Build history of the part. All positions in model axes, mm. Face numbers are marked on the shaded views. A direction names the side the tool comes from. Round coordinates to 2 decimals unless told otherwise and drop trailing zeros. Write each loop counter-clockwise with the first axis right and the second up, starting at its lowest first coordinate (ties: lowest second). Pieces come first, ordered by that corner, then holes. Notation, with made-up numbers: (17, 9) -> (41, 9) arc R9 ccw to (41, 18) -> close; hole circle Ø6 at (-3.5, 55). An arc over 180 degrees is marked (long way). Return JSON: item names as keys, results as strings.
from build123d import *


with BuildPart() as f1:
    # F0 (on Right) → F1 (revolve)
    with BuildSketch(Plane.YZ):
        with BuildLine():
            Line((-123.77214, 15), (-123.77214, 0))
            Line((-123.77214, 0), (96.22786, 0))
            Line((96.22786, 0), (96.22786, 15))
            Line((96.22786, 15), (78.22786, 15))
            ThreePointArc((78.22786, 15), (73.278113, 17.050253), (71.22786, 22))
            Line((71.22786, 22), (71.22786, 24.047213))
            ThreePointArc((71.22786, 24.047213), (69.177608, 28.996961), (64.22786, 31.047213))
            Line((64.22786, 31.047213), (-23.778022, 31.047213))
            ThreePointArc((-23.778022, 31.047213), (-33.246551, 21.403982), (-43.675041, 30))
            Line((-43.675041, 30), (-108.77214, 30))
            ThreePointArc((-108.77214, 30), (-119.378742, 25.606602), (-123.77214, 15))
        make_face()
    revolve(axis=Axis((0, 76.22786, 0), (0, 1, 0)))


solid = f1.part
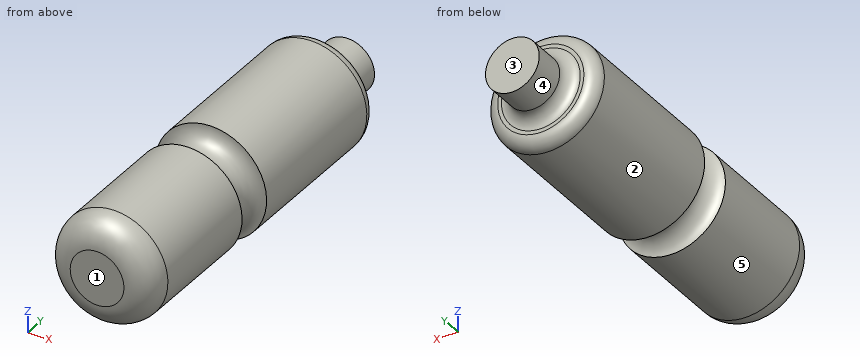
Q1. Saw through at D-D on y = -1.5. List the corners of the cut face in (x, z).
Verdict:
{"outline": "circle Ø62.09 at (0, 0)"}
Q2. Two-plate mould, pull along Z, no slides. Class the marked faces 1 and 2: +Z half, -Z half, draft (parallel to the pull), parting line (faces both ways), or undercut.
Verdict:
{"face 1": "draft", "face 2": "parting line"}
Q3. Pin check, flat tips, straight feed: pin 1 Ø1.5 at (x, y) = (-3, 31.5) entering from +Z; pin 2 Ø6 at (x, y) = (-15.5, -46.5) entering from +Z; pin 3 Ø6 at (y, z) = (16, -23.5) entering from +X. Stop position of each tip, or through.
Verdict:
{"pin 1": "stops at z = 30.97", "pin 2": "stops at z = 27.27", "pin 3": "stops at x = 23.32"}
Q4. Saw through at C-C on y = -106. List the corners of the cut face in (x, z).
Verdict:
{"outline": "circle Ø60 at (0, 0)"}
Q5. Saw through at A-A on z = 0. List the corners of the cut face in (x, y).
Verdict:
{"outline": "(-31.05, -23.78) arc R10 cw to (-30, -43.68) -> (-30, -108.77) arc R15 ccw to (-15, -123.77) -> (15, -123.77) arc R15 ccw to (30, -108.77) -> (30, -43.68) arc R10 cw to (31.05, -23.78) -> (31.05, 64.23) arc R7 ccw to (24.05, 71.23) -> (22, 71.23) arc R7 cw to (15, 78.23) -> (15, 96.23) -> (-15, 96.23) -> (-15, 78.23) arc R7 cw to (-22, 71.23) -> (-24.05, 71.23) arc R7 ccw to (-31.05, 64.23) -> close"}
Q6. Saw through at B-B on x = 0. List the corners of the cut face in (y, z), then the cut area to 3 significant figures.
Verdict:
{"outline": "(-123.77, -15) arc R15 ccw to (-108.77, -30) -> (-43.68, -30) arc R10 cw to (-23.78, -31.05) -> (64.23, -31.05) arc R7 ccw to (71.23, -24.05) -> (71.23, -22) arc R7 cw to (78.23, -15) -> (96.23, -15) -> (96.23, 15) -> (78.23, 15) arc R7 cw to (71.23, 22) -> (71.23, 24.05) arc R7 ccw to (64.23, 31.05) -> (-23.78, 31.05) arc R10 cw to (-43.68, 30) -> (-108.77, 30) arc R15 ccw to (-123.77, 15) -> close", "area": "12,300 mm²"}
Q7. 3-axis set-ups, long thin cutter, end or side, ignore diameter. For the marked faces 3, 4 and 5: which of +Z, -Z, +X, -X, +Y, -Y reach the whole face in a straight line?
Verdict:
{"face 3": "+Z, -Z, +X, -X, +Y", "face 4": "+Y", "face 5": "-Y"}
Q8. Wall check: L1, parallel to Z at x = -8, y = -20; L2, parallel to Y at x = 13, z = 23.5; L3, parallel to Y at x = 16, z = -18. Give the ranges that are in metal, low to high.
Verdict:
{"L1": "z = -30 to 30", "L2": "y = -117.96 to -42.69, -24.86 to 70.64", "L3": "y = -120.71 to -40.6, -26.95 to 71.23"}
